Work out the finished part from the listing and answer in its coordinate system (mm). A direction names the side the tool comes from. Round coordinates to 2 decimals unless told otherwise and drop trailing zeros. Order: outer loops, then holes, each group sorted by start corner. A loop starts at its lowest first (then second) coordinate and runs counter-clockwise, first axis right, second up. Notation, with made-up numbers: (24.5, 42.25) -> (78.5, 42.25) arc R27 ccw to (78.5, 64.25) -> close; hole circle Ø11 at (49, 79.25). An arc over 180 degrees is marked (long way). Use a Markdown table: item, result. Add a question column.
Item 1: For a pull along X with two mould halves and no side action, classify faces 1 (the flat face through (10, 41, -1.5)), 2 (the cylindrical face through (32.537, 0.202, -40.463)), 3 (the cylindrical face through (32.537, 0.202, 40.506)), 4 (the flat face through (20, -41, 0)) as +X half, -X half, draft (parallel to the pull), parting line (faces both ways), or undercut.
Item 2: A tool of negligible diameter and unlimited length cuts with its end or side. For faces 5 (the flat face through (10, 40, 0)), 6 (the flat face through (20, 0, -41)), 7 (the flat face through (10, -41, -1.5)), 8 (the flat face through (10, 0, 40)), 9 (the flat face through (25, -8.5, -37.4)), from which of +Z, -Z, +X, -X, +Y, -Y can it reach the whole face along a straight path? Write none if from no direction.
Item 3: A cutting plane is placed at C-C, the plane x = 6. Determine the outline of the cut face in (y, z).
Item 4: Find the intervals of material crossed by L1, parallel to Z at x = 19, y = 1; L2, parallel to X at y = 40.7, z = 0; L3, parallel to X at y = 0, z = -39.7, in increasing order. Write a range as [from, to].
Item 5: Flat-ended cylindrical pins translate along their axes: P1, Ø2, axis at x = 24.5, z = -6, coming from the -Y side; P2, Ø12, axis at x = 33, z = 8, coming from the -Y side; P3, Ø3.5, axis at x = 5.5, y = -0.5, coming from the +Z side; P4, Ø3.5, axis at x = 31, z = 0, coming from the -Y side. Find the tip coordinate at first contact, or state that the pin passes through.
Item 6: A cutting plane is placed at A-A, the plane z = 0. Determine the outline of the cut face in (x, y).
Item 7: A cutting plane is placed at D-D, the plane z = -22. Determine the outline of the cut face in (x, y).
from build123d import *

# Parameters (mm, degrees)
D_GAGEMENT_M2_51_D           = 3.1
R_P_TITION_CIRCULAIRE1_COUNT = 2
R_P_TITION_CIRCULAIRE1_ANGLE = 90
ESQUISSE5_W                  = 3
ESQUISSE5_H                  = 15
ENL_V_MAT_EXTRU_1_DEPTH      = 20
R_P_TITION_CIRCULAIRE2_COUNT = 4


with BuildPart() as part:
    # Esquisse1 → Révolution1 (revolve)
    with BuildSketch(Plane.XY):
        Polygon((0, 38.15), (25, 38.15), (25, 39), (40, 39), (40, 42), (0, 42), align=None)
    revolve(axis=Axis((0, 0, 0), (1, 0, 0)))

    # Dégagement M2.51 (through all)
    with Locations(Plane(origin=(31, 42, 0), x_dir=(0, 0, 1), z_dir=(0, 1, 0))):
        with Locations((0, 0)):
            d_gagement_m2_51 = Hole(D_GAGEMENT_M2_51_D / 2)

    # Répétition circulaire1: Dégagement M2.51 ×2 about axis
    r_p_tition_circulaire1_axis = Axis((40, 0, 0), (-1, 0, 0))
    for i in range(1, R_P_TITION_CIRCULAIRE1_COUNT):
        add(d_gagement_m2_51.rotate(r_p_tition_circulaire1_axis, i * R_P_TITION_CIRCULAIRE1_ANGLE / (R_P_TITION_CIRCULAIRE1_COUNT - 1)), mode=Mode.SUBTRACT)

    # Esquisse5 → Enlèv. mat.-Extru.1 (cut)
    with BuildSketch(Plane.ZY):
        with Locations((0, 47.5)):
            Rectangle(ESQUISSE5_W, ESQUISSE5_H)
    enl_v_mat_extru_1 = extrude(amount=-ENL_V_MAT_EXTRU_1_DEPTH, mode=Mode.SUBTRACT)

    # Répétition circulaire2: Enlèv. mat.-Extru.1 ×4 about axis
    r_p_tition_circulaire2_axis = Axis((0, 0, 0), (1, 0, 0))
    for i in range(1, R_P_TITION_CIRCULAIRE2_COUNT):
        add(enl_v_mat_extru_1.rotate(r_p_tition_circulaire2_axis, i * 360 / R_P_TITION_CIRCULAIRE2_COUNT), mode=Mode.SUBTRACT)


solid = part.part
Reported:
| question | item | result |
|---|---|---|
| 1 | face 1 | draft |
| 1 | face 2 | undercut |
| 1 | face 3 | undercut |
| 1 | face 4 | -X half |
| 2 | face 5 | -X, +Y |
| 2 | face 6 | -Z, -X |
| 2 | face 7 | -X, -Y |
| 2 | face 8 | +Z, -X |
| 2 | face 9 | +X |
| 3 | outline | (-41.97, -1.5) arc R42 ccw to (-1.5, -41.97) -> (-1.5, -40) -> (1.5, -40) -> (1.5, -41.97) arc R42 ccw to (41.97, -1.5) -> (40, -1.5) -> (40, 1.5) -> (41.97, 1.5) arc R42 ccw to (1.5, 41.97) -> (1.5, 40) -> (-1.5, 40) -> (-1.5, 41.97) arc R42 ccw to (-41.97, 1.5) -> (-40, 1.5) -> (-40, -1.5) -> close; hole circle Ø76.3 at (0, 0) |
| 4 | L1 | [-40, -38.14], [38.14, 40] |
| 4 | L2 | [20, 29.45], [32.55, 40] |
| 4 | L3 | [0, 29.45], [32.55, 40] |
| 5 | P1 | y = -41.7 |
| 5 | P2 | y = -41.95 |
| 5 | P3 | z = 41.97 |
| 5 | P4 | y = -42 |
| 6 | outline | (0, -40) -> (20, -40) -> (20, -42) -> (29.45, -42) -> (29.45, -39) -> (25, -39) -> (25, -38.15) -> (0, -38.15) -> close; (0, 38.15) -> (25, 38.15) -> (25, 39) -> (29.45, 39) -> (29.45, 42) -> (20, 42) -> (20, 40) -> (0, 40) -> close; (32.55, -42) -> (40, -42) -> (40, -39) -> (32.55, -39) -> close; (32.55, 39) -> (40, 39) -> (40, 42) -> (32.55, 42) -> close |
| 7 | outline | (0, -35.78) -> (40, -35.78) -> (40, -32.2) -> (25, -32.2) -> (25, -31.17) -> (0, -31.17) -> close; (0, 31.17) -> (25, 31.17) -> (25, 32.2) -> (40, 32.2) -> (40, 35.78) -> (0, 35.78) -> close |
